Verification items for the finished model (mm, model axes). Face numbers are marked on the shaded views. A direction names the side the tool comes from. Give positions to 0.01 mm unless a question says otherwise; leave off trailing zeros. Write item = value, one per line.
from build123d import *

# Parameters (mm, degrees)
EXTRUDE_1_DEPTH = 10
SHELL_2_T       = 5
FILLET_3_R      = 10
FILLET_4_R      = 5
SKETCH_2_R      = 2.8
EXTRUDE_2_DEPTH = 8


# Some blends are built 0.0001 mm under size
with BuildPart() as part:
    # 草图1 → 凸台-拉伸1 (new body)
    with BuildSketch(Plane(origin=(0, 0, 0), x_dir=(1, 0, 0), z_dir=(0, 1, 0))):
        with BuildLine():
            Line((-37.5, 15), (37.5, 15))
            ThreePointArc((37.5, 15), (44.571067812, 12.071067812), (47.5, 5))
            Line((47.5, 5), (47.5, -5))
            ThreePointArc((47.5, -5), (44.571067812, -12.071067812), (37.5, -15))
            Line((37.5, -15), (-37.5, -15))
            ThreePointArc((-37.5, -15), (-44.571067812, -12.071067812), (-47.5, -5))
            Line((-47.5, -5), (-47.5, 5))
            ThreePointArc((-47.5, 5), (-44.571067812, 12.071067812), (-37.5, 15))
        make_face()
    extrude(amount=EXTRUDE_1_DEPTH)

    # 抽壳2
    shell_2_openings = [part.faces().sort_by_distance(p)[0] for p in [
        (0, 0, 0),
    ]]
    offset(amount=SHELL_2_T, openings=shell_2_openings, kind=Kind.INTERSECTION)

    # 圆角3
    # the kernel refuses this fillet: 10 mm, written as the material it takes off along each edge
    with BuildSketch(Plane(origin=(37.5, 15, 5), x_dir=(1, 0, 0), z_dir=(0, 0, -1))) as fillet_3_piece_1:
        with BuildLine():
            CenterArc((15 - FILLET_3_R, FILLET_3_R), FILLET_3_R, 270, 90)
            Line((15 - FILLET_3_R, 0), (15, 0))
            Line((15, 0), (15, FILLET_3_R))
        make_face()
    revolve(axis=Axis((37.5, 15, 5), (0, -1, 0)), revolution_arc=90, mode=Mode.SUBTRACT)
    with BuildSketch(Plane(origin=(52.5, 15, 5), x_dir=(0, -1, 0), z_dir=(0, 0, -1)), Plane(origin=(-52.5, 15, -5), x_dir=(0, -1, 0), z_dir=(0, 0, 1))) as fillet_3_piece_2:
        with BuildLine():
            CenterArc((FILLET_3_R, FILLET_3_R), FILLET_3_R, 180, 90)
            Line((0, FILLET_3_R), (0, 0))
            Line((0, 0), (FILLET_3_R, 0))
        make_face()
    extrude(amount=10, mode=Mode.SUBTRACT)
    with BuildSketch(Plane(origin=(37.5, 15, -5), x_dir=(0, 0, -1), z_dir=(-1, 0, 0))) as fillet_3_piece_3:
        with BuildLine():
            CenterArc((15 - FILLET_3_R, FILLET_3_R), FILLET_3_R, 270, 90)
            Line((15 - FILLET_3_R, 0), (15, 0))
            Line((15, 0), (15, FILLET_3_R))
        make_face()
    revolve(axis=Axis((37.5, 15, -5), (0, -1, 0)), revolution_arc=90, mode=Mode.SUBTRACT)
    with BuildSketch(Plane(origin=(37.5, 15, -20), x_dir=(0, -1, 0), z_dir=(-1, 0, 0)), Plane(origin=(-37.5, 15, 20), x_dir=(0, -1, 0), z_dir=(1, 0, 0))) as fillet_3_piece_4:
        with BuildLine():
            CenterArc((FILLET_3_R, FILLET_3_R), FILLET_3_R, 180, 90)
            Line((0, FILLET_3_R), (0, 0))
            Line((0, 0), (FILLET_3_R, 0))
        make_face()
    extrude(amount=75, mode=Mode.SUBTRACT)
    with BuildSketch(Plane(origin=(-37.5, 15, -5), x_dir=(-1, 0, 0), z_dir=(0, 0, 1))) as fillet_3_piece_5:
        with BuildLine():
            CenterArc((15 - FILLET_3_R, FILLET_3_R), FILLET_3_R, 270, 90)
            Line((15 - FILLET_3_R, 0), (15, 0))
            Line((15, 0), (15, FILLET_3_R))
        make_face()
    revolve(axis=Axis((-37.5, 15, -5), (0, -1, 0)), revolution_arc=90, mode=Mode.SUBTRACT)
    with BuildSketch(Plane(origin=(-37.5, 15, 5), x_dir=(0, 0, 1), z_dir=(1, 0, 0))) as fillet_3_piece_6:
        with BuildLine():
            CenterArc((15 - FILLET_3_R, FILLET_3_R), FILLET_3_R, 270, 90)
            Line((15 - FILLET_3_R, 0), (15, 0))
            Line((15, 0), (15, FILLET_3_R))
        make_face()
    revolve(axis=Axis((-37.5, 15, 5), (0, -1, 0)), revolution_arc=90, mode=Mode.SUBTRACT)

    # 圆角4
    fillet_4_edges = [part.edges().sort_by_distance(p)[0] for p in [
        (52.5, 0, 0),
        (48.106601718, 0, 15.606601718),
        (0, 0, 20),
        (-48.106601718, 0, 15.606601718),
        (-52.5, 0, 0),
        (-48.106601718, 0, -15.606601718),
        (0, 0, -20),
        (48.106601718, 0, -15.606601718),
    ]]
    fillet(fillet_4_edges, radius=FILLET_4_R - 0.0001)  # a hair under: the kernel refuses the full size

    # 草图2 → 凸台-拉伸2 (add)
    # profile 1 of 2: a face of its own
    with BuildSketch(Plane(origin=(0, 10, 0), x_dir=(-1, 0, 0), z_dir=(0, -1, 0))):
        with Locations(Location((37, 0, 0), (0, 0, 270))):
            Circle(SKETCH_2_R)
        Polygon((34.825, -0.7), (34.825, 0.7), (36.3, 0.7), (36.3, 2.175), (37.7, 2.175), (37.7, 0.7), (39.175, 0.7), (39.175, -0.7), (37.7, -0.7), (37.7, -2.175), (36.3, -2.175), (36.3, -0.7), align=None, mode=Mode.SUBTRACT)
    # profile 2 of 2: a face of its own
    with BuildSketch(Plane(origin=(0, 10, 0), x_dir=(-1, 0, 0), z_dir=(0, -1, 0))):
        with Locations(Location((-37, 0, 0), (0, 0, 90))):
            Circle(SKETCH_2_R)
        Polygon((-37.7, 0.7), (-37.7, 2.175), (-36.3, 2.175), (-36.3, 0.7), (-34.825, 0.7), (-34.825, -0.7), (-36.3, -0.7), (-36.3, -2.175), (-37.7, -2.175), (-37.7, -0.7), (-39.175, -0.7), (-39.175, 0.7), align=None, mode=Mode.SUBTRACT)
    extrude(amount=EXTRUDE_2_DEPTH)


solid = part.part
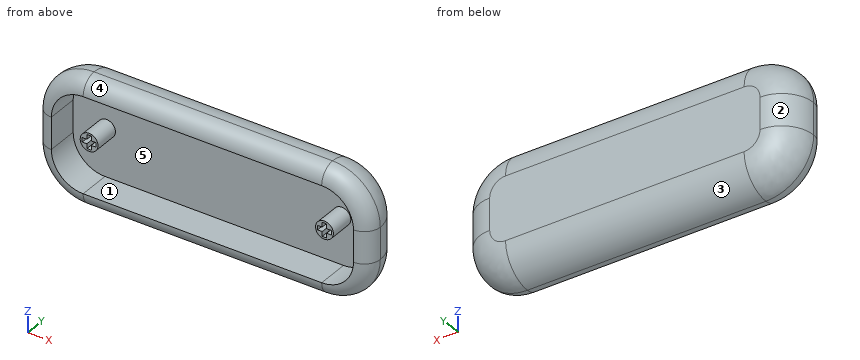
1) Material ranges on probe 1 along Z at (x, y) = (-19, 5); probe 2 along X at (y, z) = (8, 1); probe 3 along Z at (x, y) = (-34.5, 8), recorded low to high. Write a range as from..to.
From the geometry:
probe_1 = -20..-15, 15..20
probe_2 = -52.04..-47.5, -39.62..-37.7, -36.3..-34.38, 34.38..36.3, 37.7..39.62, 47.5..52.04
probe_3 = -19.54..-15, -1.26..1.26, 15..19.54
2) Depth check by flat-ended pin: P1, Ø15, axis at x = 15.5, z = -3.5, coming from the -Y side; P2, Ø10, axis at x = 40, z = -1.5, coming from the -Y side; P3, Ø1.5, axis at x = 20.5, y = 2, coming from the +Z side. Enter the tip coordinate at first touch or a pass-through.
From the geometry:
P1 = 10
P2 = 2
P3 = 19.47
3) Cross-section at B-B on y = 3. Count the separate pieces of the cut face and the enclosed holes in it, plus the area to 3 significant figures.
From the geometry:
separate_pieces = 3
enclosed_holes = 3
area = 1,160 mm^2
4) Draft check along Z on the marked faces 1, 2 and 3. Enter one of: +Z half, -Z half, draft (parallel to the pull), parting line (faces both ways), or undercut.
From the geometry:
face_1 = undercut
face_2 = draft
face_3 = -Z half
5) Tool access check on the marked faces 4 and 5. Record the directions out of +Z, -Z, +X, -X, +Y, -Y that give a thin tool (end or side, any length) a straight path to the whole face; none if there is none.
From the geometry:
face_4 = +Z, +X, -X, -Y
face_5 = -Y
